Verification items for this drawing (mm, ordinates from the low corner). A direction names the side the tool comes from. Round coordinates to 2 decimals unless told otherwise and drop trailing zeros. Loops run counter-clockwise (first coordinate to the right, second up) from the corner with the lowest first, then second, coordinate; pieces in that order, holes last. Notation, with made-up numbers: (59, 8.5) -> (116, 8.5) arc R21 cw to (116, 29.5) -> close; hole circle Ø10 at (-37.75, 52). An arc over 180 degrees is marked (long way). Use a Markdown table: item, result. Add a question column.
Q1. Sectioned sample at A-A, the plane z = 59.5. Enter the section's corners in (x, y).
Q2. Sectioned sample at B-B, the plane x = 89. Enter the section's corners in (y, z) (1 decimal), then the cut area to 3 significant figures.
Q3. Sectioned sample at C-C, the plane y = 44. Enter the section's corners in (x, z), then the cut area to 3 significant figures.
Q4. Material ranges on L1, parallel to Y at x = 81.5, z = 22; L2, parallel to Y at x = 94, z = 45.5; L3, parallel to Z at x = 62, y = 59, recorded low to high.
Q5. Gauge pin test, flat ends, axial feed: P1, Ø6, axis at x = 24, y = 69.5, coming from the +Z side; P2, Ø6, axis at x = 41.5, z = 21, coming from the +Y side. Record the tip position at first contact, or that the pin passes through.
Q6. Sectioned sample at D-D, the plane z = 7.5. Enter the section's corners in (x, y) (1 decimal).
Q7. Set-up check for the marked faces 5, 6 and 7: record each of +Z, -Z, +X, -X, +Y, -Y from which the full face is reachable in a straight line by a thin tool's end or side.
Q8. Release check for a two-part mould opening along Y. For the marked faces 1, 2, 3 and 4 record: released by +Y, released by -Y, zero draft, split by the parting line, or undercut.
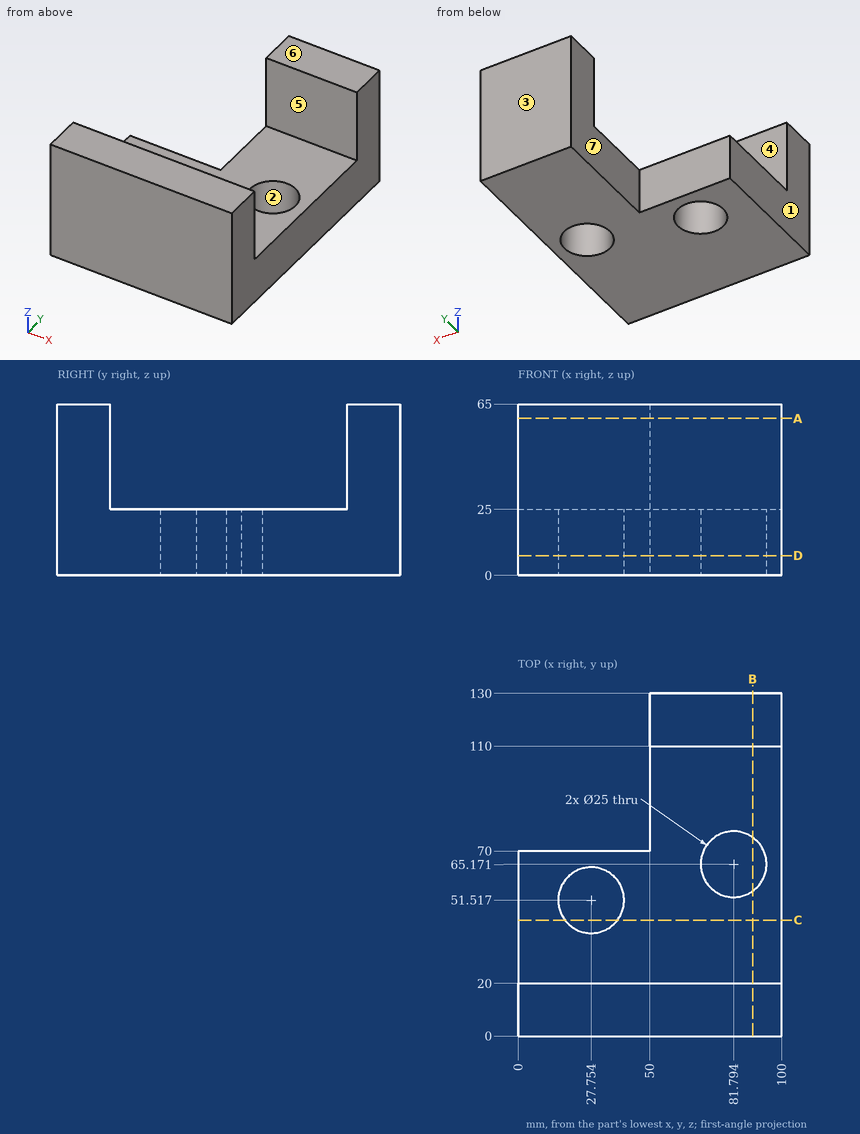
Values:
| question | item | result |
|---|---|---|
| 1 | outline | (0, 0) -> (100, 0) -> (100, 20) -> (0, 20) -> close; (50, 110) -> (100, 110) -> (100, 130) -> (50, 130) -> close |
| 2 | outline | (0, 0) -> (55, 0) -> (55, 25) -> (20, 25) -> (20, 65) -> (0, 65) -> close; (75.4, 0) -> (130, 0) -> (130, 65) -> (110, 65) -> (110, 25) -> (75.4, 25) -> close |
| 2 | area | 4,340 mm^2 |
| 3 | outline | (0, 0) -> (17.77, 0) -> (17.77, 25) -> (0, 25) -> close; (37.74, 0) -> (100, 0) -> (100, 25) -> (37.74, 25) -> close |
| 3 | area | 2,000 mm^2 |
| 4 | L1 | 0 to 52.67, 77.67 to 130 |
| 4 | L2 | 0 to 20, 110 to 130 |
| 4 | L3 | 0 to 25 |
| 5 | P1 | z = 25 |
| 5 | P2 | y = 70 |
| 6 | outline | (0, 0) -> (100, 0) -> (100, 130) -> (50, 130) -> (50, 70) -> (0, 70) -> close; hole circle Ø25 at (27.8, 51.5); hole circle Ø25 at (81.8, 65.2) |
| 7 | face 5 | +Z, +X, -X |
| 7 | face 6 | +Z, +X, -X, +Y, -Y |
| 7 | face 7 | +Z, -Z, -X, +Y |
| 8 | face 1 | zero draft |
| 8 | face 2 | undercut |
| 8 | face 3 | released by +Y |
| 8 | face 4 | undercut |
